```python
from build123d import *

# Parameters (mm, degrees)
SKETCH4_R              = 10
CUT_EXTRUDE1_DEPTH     = 76
M24_TAPPED_HOLE1_D     = 21
M24_TAPPED_HOLE1_DEPTH = 27
M24_TAPPED_HOLE1_TIP   = 6.062177826
M12_TAPPED_HOLE1_D     = 12
M12_TAPPED_HOLE1_DEPTH = 15
M12_TAPPED_HOLE1_TIP   = 3.464101615


with BuildPart() as part:
    # Sketch2 → Revolve1 (revolve)
    with BuildSketch(Plane(origin=(0, 0, 0), x_dir=(0, 0, -1), z_dir=(1, 0, 0))):
        with BuildLine():
            Line((28, 0), (88, 0))
            ThreePointArc((88, 0), (89.757359313, -4.242640687), (94, -6))
            Line((94, -6), (138, -6))
            Line((138, -6), (138, -28))
            Line((138, -28), (81, -28))
            Line((81, -28), (81, -34))
            Line((81, -34), (35, -81))
            Line((35, -81), (14, -81))
            Line((14, -81), (14, -50))
            Line((14, -50), (28, -41.917096231))
            Line((28, -41.917096231), (28, 0))
        make_face()
    revolve(axis=Axis((0, 70.454304255, 0), (0, -1, 0)))

    # Sketch4 → Cut-Extrude1 (cut, through all)
    with BuildSketch(Plane(origin=(0, -6, 0), x_dir=(1, 0, 0), z_dir=(0, 1, 0))):
        with Locations((0, 112.5)):
            Circle(SKETCH4_R)
        with Locations((97.427857926, 56.25)):
            Circle(SKETCH4_R)
        with Locations((97.427857926, -56.25)):
            Circle(SKETCH4_R)
        with Locations((0, -112.5)):
            Circle(SKETCH4_R)
        with Locations((-97.427857926, -56.25)):
            Circle(SKETCH4_R)
        with Locations((-97.427857926, 56.25)):
            Circle(SKETCH4_R)
    extrude(amount=-CUT_EXTRUDE1_DEPTH, mode=Mode.SUBTRACT)

    # M24 Tapped Hole1
    with Locations(Plane(origin=(0, 0, 0), x_dir=(1, 0, 0), z_dir=(0, 1, 0))):
        with Locations((0, -60), (0, 60)):
            Hole(M24_TAPPED_HOLE1_D / 2, depth=M24_TAPPED_HOLE1_DEPTH)
            with Locations((0, 0, -(M24_TAPPED_HOLE1_DEPTH + M24_TAPPED_HOLE1_TIP / 2))):  # 120° drill point
                Cone(0, M24_TAPPED_HOLE1_D / 2, M24_TAPPED_HOLE1_TIP, mode=Mode.SUBTRACT)

    # M12 Tapped Hole1
    with Locations(Plane(origin=(0, 0, 0), x_dir=(1, 0, 0), z_dir=(0, 1, 0))):
        with Locations((-44, 0), (44, 0)):
            Hole(M12_TAPPED_HOLE1_D / 2, depth=M12_TAPPED_HOLE1_DEPTH)
            with Locations((0, 0, -(M12_TAPPED_HOLE1_DEPTH + M12_TAPPED_HOLE1_TIP / 2))):  # 120° drill point
                Cone(0, M12_TAPPED_HOLE1_D / 2, M12_TAPPED_HOLE1_TIP, mode=Mode.SUBTRACT)


solid = part.part
```
Input: part model. Units: mm. Frame: model coordinates. A direction names the side the tool comes from. Give positions to 0.01 mm unless a question says otherwise; leave off trailing zeros. Order: outer loops, then holes, each group sorted by start corner. A loop starts at its lowest first (then second) coordinate and runs counter-clockwise, first axis right, second up. Notation, with made-up numbers: M 74,73 L 80,73 A7 cw 80,85 Z; hole C 22,28 d8. An arc over 180 degrees is marked long. Return JSON: item names as keys, results as strings.
1) Section query B-B on x = -3.5. Count the separate pieces of the cut face and the enclosed holes in it, and give its area (3 significant figures).
Taken from the geometry:
{"separate pieces": "4", "enclosed holes": "0", "area": "8,060 mm2"}
2) Contact query for flat-ended pins moving along their axis: pin 1 (12 mm diameter, centred on x = -7, y = -35, fed in from +Z); pin 2 (23 mm diameter, centred on x = 0, z = -112.5, fed in from -Y); pin 3 (4 mm diameter, centred on x = -36.5, y = -54.5, fed in from +Z); pin 4 (16 mm diameter, centred on x = -97.43, z = -56.25, fed in from +Y). Output: stop coordinate, or through.
Taken from the geometry:
{"pin 1": "stops at z = 80.99", "pin 2": "stops at y = -28", "pin 3": "stops at z = 51.6", "pin 4": "passes through"}
3) Mould query, pull axis Z, two halves, no side actions, for faces 1 (the face through (68.3, -31.042, -43.545)), 2 (the face through (-59, -28, -59)), 3 (the face through (-1.302, -16.846, 102.585)). Classes: released by +Z, released by -Z, zero draft, split by the parting line, or undercut.
Taken from the geometry:
{"face 1": "split by the parting line", "face 2": "zero draft", "face 3": "undercut"}
4) Access query for faces 4 (the face through (-38, -8, 0)), 5 (the face through (41.451, -17.154, -131.627)). Directions: +Z, -Z, +X, -X, +Y, -Y. A direction counts if a zero-diameter tool reaches every point of the face in a straight line with its end or side. Return the directions, or none.
Taken from the geometry:
{"face 4": "+Y", "face 5": "+Y, -Y"}
5) Section query C-C on x = 115.5. Output: boundary loops of the cut face in (y, z), and give its area (3 significant figures).
Taken from the geometry:
{"outline": "M -28,-75.52 L -6,-75.52 L -6,75.52 L -28,75.52 Z", "area": "3,320 mm2"}
6) Section query A-A on z = 112.5. Output: boundary loops of the cut face in (x, y), and give its area (3 significant figures).
Taken from the geometry:
{"outline": "M -79.92,-28 L -10,-28 L -10,-6 L -79.92,-6 Z; M 10,-28 L 79.92,-28 L 79.92,-6 L 10,-6 Z", "area": "3,080 mm2"}
7) Line query: L1, parallel to X at y = -11.5, z = 0.5; L2, parallel to X at y = -20, z = -56.25; L3, parallel to Y at x = -50.5, z = 102.5. Output: solid intervals per line, ascending. Write a range as [from, to].
Taken from the geometry:
{"L1": "x = [-138, -49.98], [-38.02, -28], [28, 38.02], [49.98, 138]", "L2": "x = [-126.02, -107.43], [-87.43, -9.81], [9.81, 87.43], [107.43, 126.02]", "L3": "y = [-28, -6]"}
